from build123d import *

# Parameters (mm, degrees)
F_9_64_ALLEN_DEPTH = 3.175


with BuildPart() as part:
    # Sketch1 → Revolve1 (revolve)
    with BuildSketch(Plane(origin=(0, 0, 0), x_dir=(1, 0, 0), z_dir=(0, 1, 0))):
        Polygon((0, 0), (0, 42.2656), (2.0828, 42.2656), (2.0828, 4.1656), (3.429, 4.1656), (3.429, 0), align=None)
    revolve(axis=Axis((0, 0, 0), (0, 0, -1)))

    # Sketch2 → 9-64 allen (cut)
    with BuildSketch(Plane.XY):
        Polygon((2.062222993, 0), (1.031111496, 1.7859375), (-1.031111496, 1.7859375), (-2.062222993, 0), (-1.031111496, -1.7859375), (1.031111496, -1.7859375), align=None)
    extrude(amount=-F_9_64_ALLEN_DEPTH, mode=Mode.SUBTRACT)


solid = part.part
Model file for the job. Use its own axes, mm. A direction names the side the tool comes from. Coordinates: 2 decimals unless noted, no trailing zeros. Order: outer loops, then holes, each group sorted by start corner. A loop starts at its lowest first (then second) coordinate and runs counter-clockwise, first axis right, second up. Notation, with made-up numbers: M -8,-28.5 L 32,-28.5 A19 cw 32,5.5 Z; hole C 63.25,69 d8. An arc over 180 degrees is marked long. Return JSON: item names as keys, results as strings.
1. Saw through at A-A (z = -2.5). Give the cut face in (x, y), and give its area (3 significant figures).
Ans:
{"outline": "C 0,0 d6.86; hole M -2.06,0 L -1.03,-1.79 L 1.03,-1.79 L 2.06,0 L 1.03,1.79 L -1.03,1.79 Z", "area": "25.9 mm^2"}
2. Saw through at B-B (x = 0). Give the cut face in (y, z) (3 decimals), and give its area (3 significant figures).
Ans:
{"outline": "M -3.429,-4.166 L -2.083,-4.166 L -2.083,-42.266 L 2.083,-42.266 L 2.083,-4.166 L 3.429,-4.166 L 3.429,0 L 1.786,0 L 1.786,-3.175 L -1.786,-3.175 L -1.786,0 L -3.429,0 Z", "area": "176 mm^2"}
3. Saw through at D-D (z = -34). Give the cut face in (x, y).
Ans:
{"outline": "C 0,0 d4.17"}
4. Tool access for faces 4 (the face through (0.05, 2.24, -4.166)), 5 (the face through (1.554, 0.88, -1.565)), 6 (the face through (1.5, 1.5, 0)): list every direction of +Z, -Z, +X, -X, +Y, -Y with a clear straight run to the whole face (end or side of a thin tool).
Ans:
{"face 4": "-Z", "face 5": "+Z", "face 6": "+Z, +X, -X, +Y, -Y"}
5. Drill centre lines: probe 1 along Z at (x, y) = (-1, -0.75) (3 decimals); probe 2 along Y at (x, z) = (-0.25, -28.5); probe 3 along X at (y, z) = (-1.5, -1.5). Where is each one in solid material? Low to high.
Ans:
{"probe 1": "-42.266 to -3.175", "probe 2": "-2.07 to 2.07", "probe 3": "-3.08 to -1.2, 1.2 to 3.08"}
6. Pull direction Y, two halves, no side cores. Call faces 1 (the face through (0, 0, -42.266)), 2 (the face through (-0.74, 3.35, -2.05)), 3 (the face through (-1.539, 0.905, -1.565)): +Y half, -Y half, draft (parallel to the pull), parting line (faces both ways), or undercut.
Ans:
{"face 1": "draft", "face 2": "parting line", "face 3": "undercut"}
7. Flat gauge pins, fed straight in: pin 1 (3 mm diameter, centred on y = -2, z = -35.5, fed in from -X); pin 2 (1 mm diameter, centred on x = 0.5, z = -13.5, fed in from +Y); pin 3 (1 mm diameter, centred on x = 0.5, z = -33.5, fed in from -Y). Where does each tip first touch, or does it go through?
Ans:
{"pin 1": "x = -2.02", "pin 2": "y = 2.08", "pin 3": "y = -2.08"}
8. Saw through at C-C (y = 1.25). Give the cut face in (x, z) (3 decimals), and give its area (3 significant figures).
Ans:
{"outline": "M -3.193,-4.166 L -1.666,-4.166 L -1.666,-42.266 L 1.666,-42.266 L 1.666,-4.166 L 3.193,-4.166 L 3.193,0 L 1.341,0 L 1.341,-3.175 L -1.341,-3.175 L -1.341,0 L -3.193,0 Z", "area": "145 mm^2"}
